Autodesk Inventor part; units mm, degrees
ref_plane "YZ Plane" through (0, 0, 0) normal (1, 0, 0) x (0, 1, 0)
ref_plane "XZ Plane" through (0, 0, 0) normal (0, 1, 0) x (-1, 0, 0)
ref_plane "XY Plane" through (0, 0, 0) normal (0, 0, 1) x (1, 0, 0)
sketch "Sketch1" plane through (0, 0, 0) normal (0, 0, 1) x (1, 0, 0)
  line L0 (-1000, 1000) -> (1000, 1000)
  line L1 (1000, 1000) -> (1000, -1000)
  line L2 (1000, -1000) -> (-1000, -1000)
  line L3 (-1000, -1000) -> (-1000, 1000)
  line L4 (-1000, 1000) -> (1000, -1000) construction
  line L5 (1000, 1000) -> (-1000, -1000) construction
  point P0 (0, 0)
  dimension "d0" = 2000
  dimension "d1" = 2000
extrude "Extrusion1" add sketch "Sketch1" along normal blind 200
sketch "Sketch2" plane through (0, 0, 200) normal (0, 0, 1) x (1, 0, 0)
  circle A0 centre (-746.6113, 699.1613) radius 13.5
  point P0 (0, 0)
  dimension "d4" = 27
extrude "Extrusion2" add sketch "Sketch2" along normal blind 200
pattern_sketch "Sketch Driven Pattern1" of "Extrusion2" from (-746.6113, 699.1613, 200) copies at (-368.7113, 600.7756, 200) at (540.698, 695.0149, 200) at (649.0732, 461.7726, 200) at (705.6168, 136.647, 200) at (649.0732, -155.4949, 200) at (500.6463, -459.4166, 200) at (189.6566, -697.3709, 200) at (-253.2681, -739.7786, 200) at (-385.2032, -527.7401, 200) at (81.2814, -296.8538, 200) at (-422.8989, 376.9572, 200) at (-592.5297, 101.3073, 200) at (-700.9049, -56.5436, 200) at (-893.617, 526.0067, 200) at (-905.6018, 376.9572, 200)
sketch "Sketch3" plane through (0, 0, 200) normal (0, 0, 1) x (1, 0, 0)
  point P0 (-368.7113, 600.7756)
  point P1 (175.5207, 631.4034)
  point P2 (540.698, 695.0149)
  point P3 (649.0732, 461.7726)
  point P4 (705.6168, 136.647)
  point P5 (649.0732, -155.4949)
  point P6 (500.6463, -459.4166)
  point P7 (189.6566, -697.3709)
  point P8 (-253.2681, -739.7786)
  point P9 (-385.2032, -527.7401)
  point P10 (81.2814, -296.8538)
  point P11 (-422.8989, 376.9572)
  point P12 (-592.5297, 101.3073)
  point P13 (-700.9049, -56.5436)
  point P14 (-893.617, 526.0067)
  point P15 (-905.6018, 376.9572)
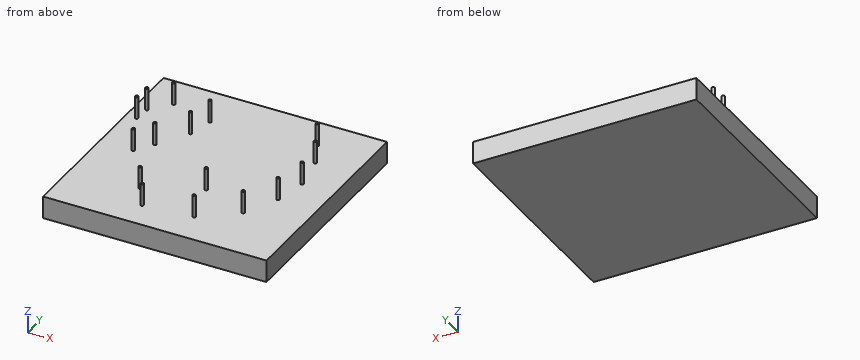
Input: part model. Units: mm. Frame: model coordinates. Coordinates: 2 decimals unless noted, no trailing zeros. Order: outer loops, then holes, each group sorted by start corner. A loop starts at its lowest first (then second) coordinate and runs counter-clockwise, first axis right, second up. Notation, with made-up numbers: M 87,30 L 111,30 A30 cw 111,56 Z; hole C 3.25,72.5 d11. An arc over 180 degrees is marked long. One line per question, with ' | ' between items.
Item 1: Section B-B (y = 792.5). Output: boundary loops of the cut face in (x, z).
Geometry results:
outline: M -1000,0 L 1000,0 L 1000,200 L -1000,200 Z
Item 2: Ray query, line 1 along Z through (x, y) = (919.5, -378); line 2 along Y through (x, z) = (-693, 226); line 3 along X through (y, z) = (-688, 342). Return the intervals inside material, ascending.
Geometry results:
line 1: z = 0 to 200 | line 2: y = -67.49 to -45.6 | line 3: x = 179.94 to 199.37
Item 3: Section A-A (z = 298). Give the number of separate pieces and of enclosed holes in the cut face, then the cut area to 3 significant figures.
Geometry results:
separate pieces: 16 | enclosed holes: 0 | area: 9,160 mm^2
